The model under review builds one solid part; all positions refer to its coordinate system, in mm. Face numbers are marked on the shaded views. A direction names the side the tool comes from. Round coordinates to 2 decimals unless told otherwise and drop trailing zeros. Loops run counter-clockwise (first coordinate to the right, second up) from the corner with the lowest first, then second, coordinate; pieces in that order, holes last. Notation, with made-up numbers: M 0.5,75.25 L 39.5,75.25 A23 cw 39.5,102.25 Z; hole C 8.25,80.5 d8. An arc over 180 degrees is marked long. Use a Markdown table: item, result. Add a question column.
Autodesk Inventor part; units mm, degrees
ref_plane "YZ Plane" through (0, 0, 0) normal (1, 0, 0) x (0, 1, 0)
ref_plane "XZ Plane" through (0, 0, 0) normal (0, 1, 0) x (-1, 0, 0)
ref_plane "XY Plane" through (0, 0, 0) normal (0, 0, 1) x (1, 0, 0)
sketch "Sketch1" plane through (0, 0, 0) normal (0, 1, 0) x (-1, 0, 0)
  line L0 (0, 0) -> (15, 0)
  line L1 (15, 0) -> (15, 34)
  line L2 (15, 34) -> (0, 34)
  line L3 (0, 34) -> (0, 0)
  line L4 (7.5, 34) -> (7.5, 36.5)
  line L5 (7.5, 36.5) -> (7.5, 47.61)
  circle A0 centre (7.5, 47.61) radius 11.11
  circle A1 centre (7.5, 47.61) radius 13.61
  line L6 (7.5, 47.61) -> (19.2866, 54.415)
  line L7 (7.5, 47.61) -> (21.11, 47.61) construction
  line L8 (7.5, 47.61) -> (-4.2866, 54.415)
  line L9 (7.5, 47.61) -> (21.11, 47.61) construction
  line L10 (15, 34) -> (18.5355, 37.5355)
  line L11 (15, 34) -> (20, 34) construction
  line L12 (18.5355, 37.5355) -> (18.5355, 39.6445)
  line L13 (0, 34) -> (-3.5355, 37.5355)
  line L14 (-3.5355, 37.5355) -> (-3.5355, 39.6445)
  point P0 (17.1215, 53.165)
  point P1 (-2.1215, 53.165)
  dimension "d0" = 15
  dimension "d1" = 34
  dimension "d2" = 2.5
  dimension "d3" = 11.11
  dimension "d4" = 30
  dimension "d5" = 150
  dimension "d6" = 5
  dimension "d7" = 45
extrude "Extrusion1" add sketch "Sketch1" along normal blind 15 contours L3 L2 L1 L0 | L13 L14 A1 L2 | L2 A1 L12 L10 | A1 L8 A0 L4 | L4 A0 L6 A1
equation "\"d8\" = d0"
properties part number "motor holder"
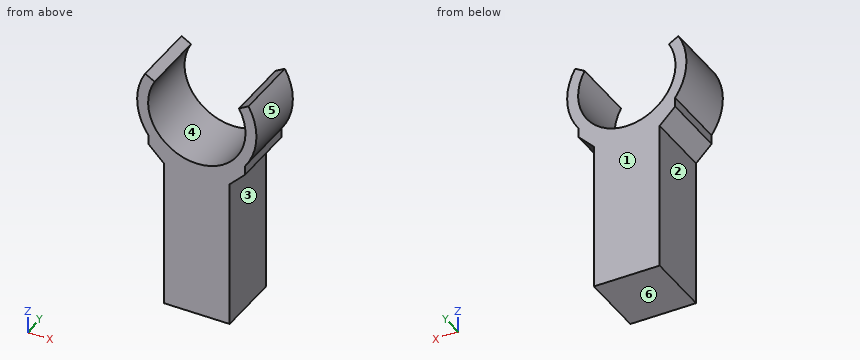
(1) Insertion check: pin 1 Ø2.5 at (y, z) = (10, 38.5) entering from +X; pin 2 Ø6 at (x, y) = (-14.5, 8.5) entering from +Z; pin 3 Ø2 at (y, z) = (7.5, 12) entering from +X. Each pin has a flat end and moves straight along its axis. Give the tip position at first contact, or say it passes through.
(2) To check wall thickness, follow probe 1 along X at (y, z) = (6.75, 47.61); probe 2 along X at (y, z) = (3.5, 25.5); probe 3 along Z at (x, y) = (-7.5, 7.5). State the ranges of each line that lie inside material, in increasing order.
(3) Draft analysis for pull direction Z (two halves, no side actions). For the marked faces 3, 4, 5 and 6, state which applies: released by +Z, released by -Z, zero draft, split by the parting line, or undercut.
(4) For the marked faces 1 and 2, list the 3-axis set-ups (+Z, -Z, +X, -X, +Y, -Y) from which the entire face can be reached by the end or side of a thin tool; tool diameter is ignored.
(5) Consider section D-D, the plane z = 42. Give the boundary of the cut face in (x, y), then the cut area to 3 significant figures.
(6) Consider section A-A, the plane z = 47.61. Give the boundary of the cut face in (x, y).
(7) Consider section B-B, the plane x = -7.5. Give the boundary of the cut face in (y, z), then the cut area to 4 significant figures.
(8) Consider section C-C, the plane y = 3.75. Give the boundary of the cut face in (x, z) (1 decimal), then the cut area to 3 significant figures.
Found:
| question | item | result |
|---|---|---|
| 1 | pin 1 | stops at x = 3.61 |
| 1 | pin 2 | stops at z = 53.38 |
| 1 | pin 3 | stops at x = 0 |
| 2 | probe 1 | x = -21.11 to -18.61, 3.61 to 6.11 |
| 2 | probe 2 | x = -15 to 0 |
| 2 | probe 3 | z = 0 to 36.5 |
| 3 | face 3 | zero draft |
| 3 | face 4 | undercut |
| 3 | face 5 | split by the parting line |
| 3 | face 6 | released by -Z |
| 4 | face 1 | +Z, -Z, +X, -X, +Y |
| 4 | face 2 | -Z, -X, +Y, -Y |
| 5 | outline | M -19.9,0 L -17.09,0 L -17.09,15 L -19.9,15 Z; M 2.09,0 L 4.9,0 L 4.9,15 L 2.09,15 Z |
| 5 | area | 84.3 mm^2 |
| 6 | outline | M -21.11,0 L -18.61,0 L -18.61,15 L -21.11,15 Z; M 3.61,0 L 6.11,0 L 6.11,15 L 3.61,15 Z |
| 7 | outline | M 0,0 L 15,0 L 15,36.5 L 0,36.5 Z |
| 7 | area | 547.5 mm^2 |
| 8 | outline | M -19.3,54.4 A13.6 ccw -18.5,39.6 L -18.5,37.5 L -15,34 L -15,0 L 0,0 L 0,34 L 3.5,37.5 L 3.5,39.6 A13.6 ccw 4.3,54.4 L 2.1,53.2 A11.1 cw long -17.1,53.2 Z |
| 8 | area | 664 mm^2 |
